Verification items for this drawing (mm, ordinates from the low corner). Round coordinates to 2 decimals unless told otherwise and drop trailing zeros. Loops run counter-clockwise (first coordinate to the right, second up) from the corner with the lowest first, then second, coordinate; pieces in that order, holes last. Notation, with made-up numbers: M 11.5,64.25 L 49.5,64.25 A26 cw 49.5,95.25 Z; hole C -9.75,-30 d3. An arc over 180 degrees is marked long. Answer as CSV lines item,"result".
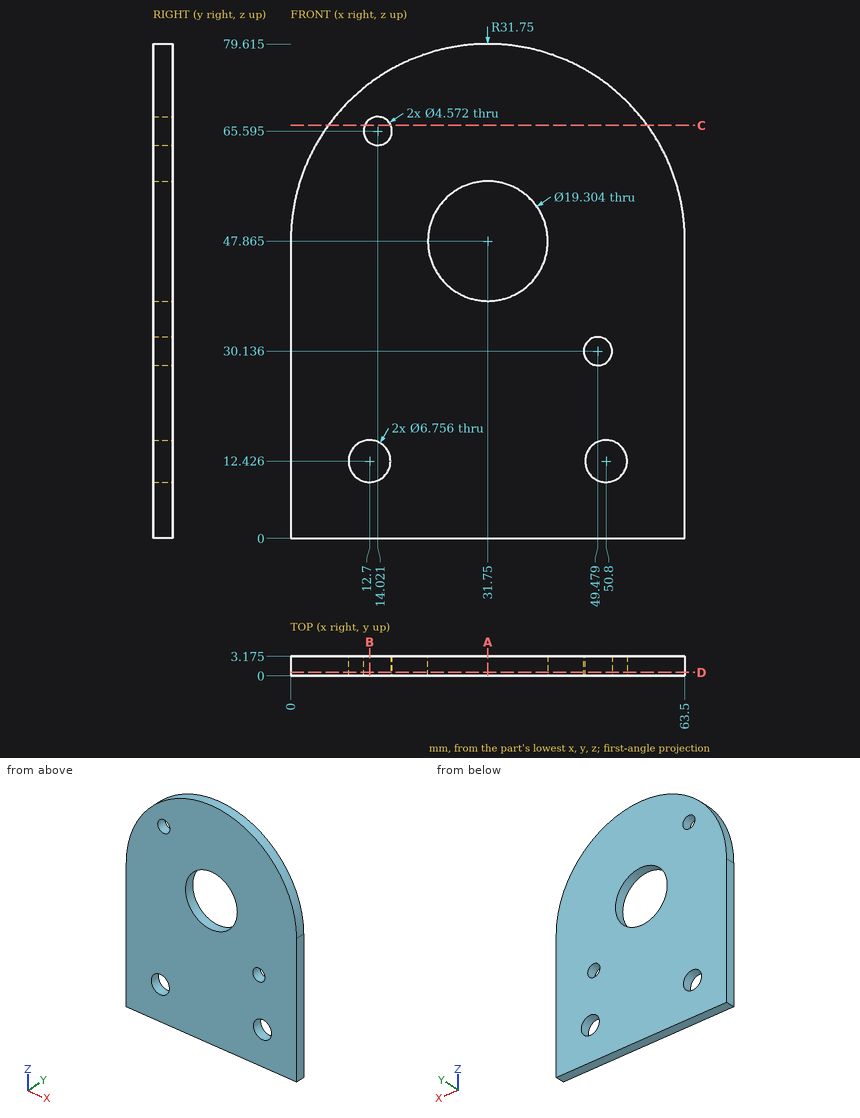
1) Section check A-A (x = 31.75). Record the cut outline in (y, z) (1 decimal).
Here are the results:
outline,"M 0,0 L 3.2,0 L 3.2,38.2 L 0,38.2 Z; M 0,57.5 L 3.2,57.5 L 3.2,79.6 L 0,79.6 Z"
2) Section check B-B (x = 12.7). Record the cut outline in (y, z) (1 decimal), plus the area to 3 significant figures.
Here are the results:
outline,"M 0,0 L 3.2,0 L 3.2,9 L 0,9 Z; M 0,15.8 L 3.2,15.8 L 3.2,63.7 L 0,63.7 Z; M 0,67.5 L 3.2,67.5 L 3.2,73.3 L 0,73.3 Z"
area,"199 mm^2"
3) Section check C-C (z = 66.5). Record the cut outline in (x, y) (1 decimal), plus the area to 3 significant figures.
Here are the results:
outline,"M 6,0 L 11.9,0 L 11.9,3.2 L 6,3.2 Z; M 16.1,0 L 57.5,0 L 57.5,3.2 L 16.1,3.2 Z"
area,"150 mm^2"
4) Go/stop test with a flat-tipped pin: pin 1 (5.5 mm diameter, centred on x = 14.02, z = 65.59, fed in from -Y). Record where the tip stops, or that it passes through.
Here are the results:
pin 1,"stops at y = 0"
5) Section check D-D (y = 0.6). State how many separate pieces and enclosed holes the cut face has, plus the area to 3 significant figures.
Here are the results:
separate pieces,"1"
enclosed holes,"5"
area,"4,230 mm^2"
6) Material ranges on probe 1 along X at (y, z) = (0.6, 10); probe 2 along Z at (x, y) = (13, 0.2); probe 3 along X at (y, z) = (2.6, 14), recorded low to high.
Here are the results:
probe 1,"x = 0 to 10.35, 15.05 to 48.45, 53.15 to 63.5"
probe 2,"z = 0 to 9.06, 15.79 to 63.55, 67.64 to 73.49"
probe 3,"x = 0 to 9.71, 15.69 to 47.81, 53.79 to 63.5"
